Drawing for the job (mm, zero at the part's lowest x, y, z). Coordinates: 2 decimals unless noted, no trailing zeros. Loops run counter-clockwise (first coordinate to the right, second up) from the corner with the lowest first, then second, coordinate; pieces in that order, holes last. Notation, with made-up numbers: (22.25, 47.5) - (40.25, 47.5) arc R18 ccw to (40.25, 51.5) - close; hole circle Ø1 at (-26.5, 75). An arc over 180 degrees is marked (long way). One line per item, written item: value.
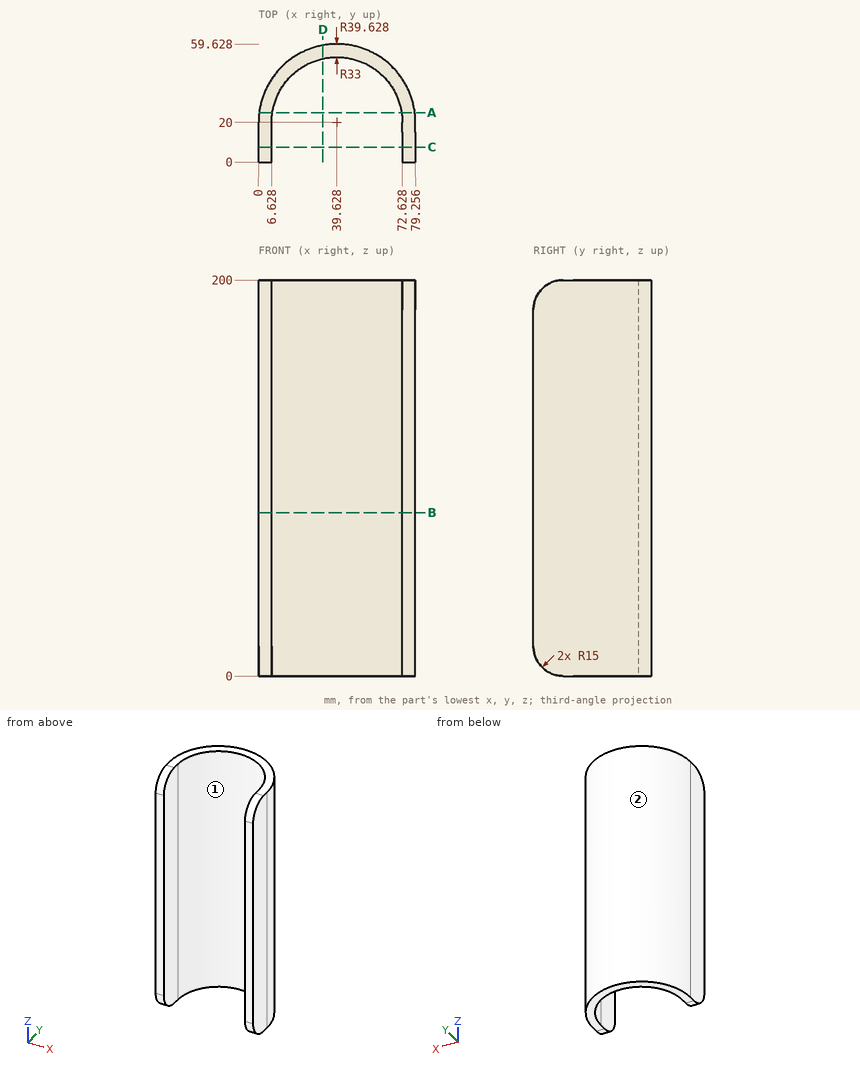
Item 1: Drop flat-ended pins along their axis: P1, Ø3, axis at x = 35, z = 56.5, coming from the +Y side; P2, Ø12, axis at y = 41.5, z = 20.5, coming from the +X side; P3, Ø1.5, axis at y = 44.5, z = 77.5, coming from the +X side; P4, Ø12, axis at x = 13.5, y = 31.5, coming from the +Z side. Give the stop position or say it passes through.
Check result:
P1: stops at y = 59.5
P2: stops at x = 76.1
P3: stops at x = 71.35
P4: stops at z = 200
Item 2: Cut at C-C, the plane y = 7.5. Write the cut outline in (x, z).
Check result:
outline: (0, 2.01) - (6.63, 2.01) - (6.63, 197.99) - (0, 197.99) - close; (72.63, 2.01) - (79.26, 2.01) - (79.26, 197.99) - (72.63, 197.99) - close
Item 3: Pull direction X, two halves, no side cores. Call the marked faces 1 and 2: released by +X, released by -X, zero draft, split by the parting line, or undercut.
Check result:
face 1: undercut
face 2: split by the parting line
Item 4: Cut at B-B, the plane z = 82.5. Write the cut outline in (x, y).
Check result:
outline: (0, 0) - (6.63, 0) - (6.63, 20) arc R33 cw to (72.63, 20) - (72.63, 0) - (79.26, 0) - (79.26, 20) arc R39.63 ccw to (0, 20) - close
Item 5: Cut at A-A, the plane y = 25. Write the cut outline in (x, z).
Check result:
outline: (0.32, 0) - (7.01, 0) - (7.01, 200) - (0.32, 200) - close; (72.25, 0) - (78.94, 0) - (78.94, 200) - (72.25, 200) - close
Item 6: Cut at D-D, the plane x = 32.5. Write the cut outline in (y, z), then the cut area to 3 significant figures.
Check result:
outline: (52.22, 0) - (58.98, 0) - (58.98, 200) - (52.22, 200) - close
area: 1,350 mm^2
Item 7: Probe probe 1 along X at (y, z) = (12, 84); probe 2 along Y at (x, z) = (39, 28); probe 3 along X at (y, z) = (39, 178). List the from-to ranges inside material, lowest first. Write a range as from..to.
Check result:
probe 1: x = 0..6.63, 72.63..79.26
probe 2: y = 52.99..59.62
probe 3: x = 4.85..12.65, 66.61..74.4
